CAD build for the part. Positions are in the model's coordinates, mm. Round coordinates to 2 decimals unless told otherwise and drop trailing zeros. Loops run counter-clockwise (first coordinate to the right, second up) from the corner with the lowest first, then second, coordinate; pieces in that order, holes last.
```python
from build123d import *

# Parameters (mm, degrees)
F0_W     = 65
F0_H     = 65
F1_DEPTH = 3
F2_R     = 5
F4_D     = 5.5
F6_D     = 7.1


with BuildPart() as f1:
    # F0 (on Top) → F1 (new body)
    with BuildSketch(Plane.XY):
        Rectangle(F0_W, F0_H)
    extrude(amount=F1_DEPTH)

    # F2
    f2_edges = [f1.edges().sort_by_distance(p)[0] for p in [
        (-32.5, 32.5, 1.5),
        (32.5, 32.5, 1.5),
        (32.5, -32.5, 1.5),
        (-32.5, -32.5, 1.5),
    ]]
    fillet(f2_edges, radius=F2_R)

    # F4 (through all)
    with Locations(Plane.XY.offset(3)):
        with Locations((-22.7, 20), (-22.7, -20), (0, -20), (0, 20), (-22.7, 0), (0, 0)):
            Hole(F4_D / 2)

    # F6 (through all)
    with Locations(Plane.XY.offset(3)):
        with Locations((22.7, 20), (22.7, -20), (22.7, 0)):
            Hole(F6_D / 2)


solid = f1.part
```
Item 1: Cut at B-B, the plane y = -20. Give the cut face in (x, z), plus the area to 3 significant figures.
Answers follow:
outline: (-32.5, 0) - (-25.45, 0) - (-25.45, 3) - (-32.5, 3) - close; (-19.95, 0) - (-2.75, 0) - (-2.75, 3) - (-19.95, 3) - close; (2.75, 0) - (19.15, 0) - (19.15, 3) - (2.75, 3) - close; (26.25, 0) - (32.5, 0) - (32.5, 3) - (26.25, 3) - close
area: 141 mm2
Item 2: Flat gauge pin, fed straight in: P1, Ø4.5, axis at x = 0, y = 20, coming from the -Z side. Where does the tip first touch, or does it go through?
Answers follow:
P1: passes through
Item 3: Cut at C-C, the plane z = 1.25. State how many separate pieces and enclosed holes the cut face has, plus the area to 3 significant figures.
Answers follow:
separate pieces: 1
enclosed holes: 9
area: 3,940 mm2
Item 4: Cut at A-A, the plane x = -22.7. Give the cut face in (y, z), plus the area to 4 significant figures.
Answers follow:
outline: (-32.5, 0) - (-22.75, 0) - (-22.75, 3) - (-32.5, 3) - close; (-17.25, 0) - (-2.75, 0) - (-2.75, 3) - (-17.25, 3) - close; (2.75, 0) - (17.25, 0) - (17.25, 3) - (2.75, 3) - close; (22.75, 0) - (32.5, 0) - (32.5, 3) - (22.75, 3) - close
area: 145.5 mm2
Item 5: Two-plate mould, pull along Y, no slides. Class faces 1 (the cylindrical face through (0.596, -2.685, 1.479)), 2 (the flat face through (0, 32.5, 1)), 3 (the flat face through (-32.5, 0, 1)): released by +Y, released by -Y, zero draft, split by the parting line, or undercut.
Answers follow:
face 1: undercut
face 2: released by +Y
face 3: zero draft
Item 6: Probe line 1 (Y direction, x = 0, z = 2.45); line 2 (X direction, y = -22, z = 0.8); line 3 (Y direction, x = 22.7, z = 0.6). List the from-to ranges inside material, lowest first.
Answers follow:
line 1: y = -32.5 to -22.75, -17.25 to -2.75, 2.75 to 17.25, 22.75 to 32.5
line 2: x = -32.5 to -24.59, -20.81 to -1.89, 1.89 to 19.77, 25.63 to 32.5
line 3: y = -32.5 to -23.55, -16.45 to -3.55, 3.55 to 16.45, 23.55 to 32.5
